Read the model definition and answer for the solid it produces. Units are mm, in the model's axes. Face numbers are marked on the shaded views. A direction names the side the tool comes from. Coordinates: 2 decimals unless noted, no trailing zeros. Order: outer loops, then holes, each group sorted by start corner. A loop starts at its lowest first (then second) coordinate and runs counter-clockwise, first axis right, second up. Notation, with made-up numbers: (64.25, 49) - (89.25, 49) arc R16 ccw to (89.25, 58) - close; hole circle Ø6 at (-22.5, -0.75). An arc over 180 degrees is marked (long way). Write item = value, one per line.
from build123d import *

# Parameters (mm, degrees)
F0_W      = 25.4
F0_H      = 25.4
F1_DEPTH  = 76.2
F2_W      = 5.08
F2_H      = 7.62
F3_DEPTH  = 25.4
F4_W      = 76.2
F4_H      = 25.4
F4_W_2    = 71.12
F4_H_2    = 15.24
F5_DEPTH  = 2.54
F6_W      = 76.2
F6_H      = 25.4
F6_W_2    = 71.12
F6_H_2    = 15.24
F7_DEPTH  = 2.54
F8_W      = 5.08
F8_H      = 7.62
F8_W_2    = 2.54
F8_W_3    = 3.81
F9_DEPTH  = 25.4
F10_W     = 7.62
F10_H     = 12.7
F11_DEPTH = 25.4
F12_W     = 2.54
F12_H     = 71.12
F13_DEPTH = 2.54
F14_W     = 71.12
F14_H     = 15.24
F15_DEPTH = 2.54
F16_W     = 12.7
F16_H     = 7.62
F17_DEPTH = 8.89
F18_W     = 12.7
F18_H     = 7.62
F19_DEPTH = 8.89
F20_W     = 12.7
F20_H     = 7.62
F21_DEPTH = 8.89
F22_W     = 20.32
F22_H     = 22.0218
F22_H_2   = 22.013333
F22_H_3   = 22.004867
F23_DEPTH = 20.32
F25_W     = 76.2
F25_H     = 2.54
F26_DEPTH = 2.54
F27_W     = 2.54
F27_H     = 76.2
F28_DEPTH = 2.54


with BuildPart() as f1:
    # F0 (on Front) → F1 (new body)
    with BuildSketch(Plane.XZ):
        with Locations((12.7, 12.7)):
            Rectangle(F0_W, F0_H)
    extrude(amount=F1_DEPTH)

    # F2 (on face) → F3 (cut)
    with BuildSketch(Plane(origin=(0, 0, 0), x_dir=(0, -1, 0), z_dir=(-1, 0, 0))):
        with Locations((7.62, 12.7)):
            Rectangle(F2_W, F2_H)
        with Locations((38.1, 12.7)):
            Rectangle(F2_W, F2_H)
        with Locations((68.58, 12.7)):
            Rectangle(F2_W, F2_H)
    extrude(amount=-F3_DEPTH, mode=Mode.SUBTRACT)

    # F4 (on face) → F5 (join)
    with BuildSketch(Plane(origin=(0, 0, 0), x_dir=(0, -1, 0), z_dir=(-1, 0, 0))):
        with Locations((38.1, 12.7)):
            Rectangle(F4_W, F4_H)
        with Locations((38.1, 12.7)):
            Rectangle(F4_W_2, F4_H_2, mode=Mode.SUBTRACT)
    extrude(amount=F5_DEPTH)

    # F6 (on face) → F7 (join)
    with BuildSketch(Plane.YZ.offset(25.4)):
        with Locations((-38.1, 12.7)):
            Rectangle(F6_W, F6_H)
        with Locations((-38.1, 12.7)):
            Rectangle(F6_W_2, F6_H_2, mode=Mode.SUBTRACT)
    extrude(amount=F7_DEPTH)

    # F8 (on face) → F9 (cut)
    with BuildSketch(Plane(origin=(0, 0, 0), x_dir=(0, -1, 0), z_dir=(-1, 0, 0))):
        with Locations((12.7, 12.7)):
            Rectangle(F8_W, F8_H)
        with Locations((3.81, 12.7)):
            Rectangle(F8_W_2, F8_H)
        with Locations((33.655, 12.7)):
            Rectangle(F8_W_3, F8_H)
        with Locations((42.545, 12.7)):
            Rectangle(F8_W_3, F8_H)
        with Locations((63.5, 12.7)):
            Rectangle(F8_W, F8_H)
        with Locations((72.39, 12.7)):
            Rectangle(F8_W_2, F8_H)
    extrude(amount=-F9_DEPTH, mode=Mode.SUBTRACT)

    # F10 (on face) → F11 (cut)
    with BuildSketch(Plane(origin=(0, 0, 0), x_dir=(1, 0, 0), z_dir=(0, 0, -1))):
        with Locations((12.7, 8.89)):
            Rectangle(F10_W, F10_H)
        with Locations((12.7, 38.1)):
            Rectangle(F10_W, F10_H)
        with Locations((12.7, 67.31)):
            Rectangle(F10_W, F10_H)
    extrude(amount=-F11_DEPTH, mode=Mode.SUBTRACT)

    # F12 (on face) → F13 (join)
    with BuildSketch(Plane(origin=(0, 0, 0), x_dir=(1, 0, 0), z_dir=(0, 0, -1))):
        Polygon((0, 76.2), (0, 73.66), (2.54, 73.66), (22.86, 73.66), (25.4, 73.66), (25.4, 76.2), align=None)
        with Locations((1.27, 38.1)):
            Rectangle(F12_W, F12_H)
        with Locations((24.13, 38.1)):
            Rectangle(F12_W, F12_H)
        Polygon((2.54, 2.54), (0, 2.54), (0, 0), (25.4, 0), (25.4, 2.54), (22.86, 2.54), align=None)
    extrude(amount=F13_DEPTH)

    # F14 (on face) → F15 (join)
    with BuildSketch(Plane(origin=(0, 0, 0), x_dir=(0, -1, 0), z_dir=(-1, 0, 0))):
        with Locations((38.1, 12.7)):
            Rectangle(F14_W, F14_H)
    extrude(amount=F15_DEPTH)

    # F16 (on face) → F17 (join)
    with BuildSketch(Plane.YZ):
        with Locations((-38.1, 12.7)):
            Rectangle(F16_W, F16_H)
    extrude(amount=F17_DEPTH)

    # F18 (on face) → F19 (join)
    with BuildSketch(Plane.YZ):
        with Locations((-67.31, 12.7)):
            Rectangle(F18_W, F18_H)
    extrude(amount=F19_DEPTH)

    # F20 (on face) → F21 (join)
    with BuildSketch(Plane.YZ):
        with Locations((-8.89, 12.7)):
            Rectangle(F20_W, F20_H)
    extrude(amount=F21_DEPTH)

    # F22 (on face) → F23 (cut)
    with BuildSketch(Plane.XY.offset(25.4)):
        with Locations((12.7, -13.5509)):
            Rectangle(F22_W, F22_H)
        with Locations((12.7, -38.108466)):
            Rectangle(F22_W, F22_H_2)
        with Locations((12.7, -62.657567)):
            Rectangle(F22_W, F22_H_3)
    extrude(amount=-F23_DEPTH, mode=Mode.SUBTRACT)

    # F25 (on face) → F26 (join)
    with BuildSketch(Plane(origin=(0, 0, 0), x_dir=(0, -1, 0), z_dir=(-1, 0, 0))):
        with Locations((38.1, -1.27)):
            Rectangle(F25_W, F25_H)
    extrude(amount=F26_DEPTH)

    # F27 (on face) → F28 (join)
    with BuildSketch(Plane(origin=(0, 0, 0), x_dir=(1, 0, 0), z_dir=(0, 0, -1))):
        with Locations((26.67, 38.1)):
            Rectangle(F27_W, F27_H)
    extrude(amount=F28_DEPTH)


solid = f1.part
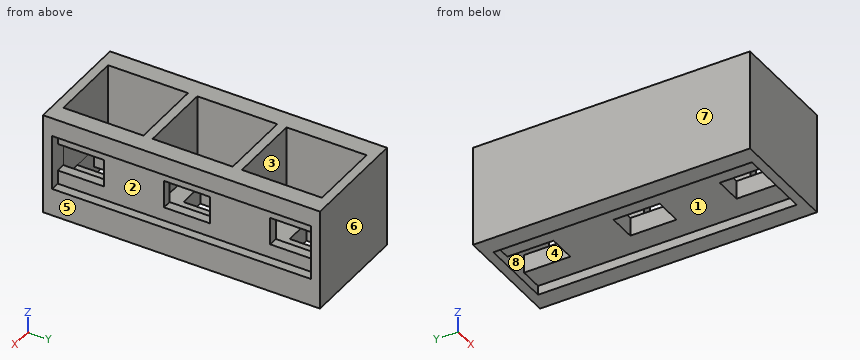
1) The part is cut by section C-C (y = -41). Determine the outline of the cut face in (x, z), and give its area (3 significant figures).
Returned:
outline = (-2.54, -2.54) - (2.54, -2.54) - (2.54, 0) - (8.89, 0) - (8.89, 5.08) - (2.54, 5.08) - (2.54, 25.4) - (-2.54, 25.4) - close; (16.51, 0) - (22.86, 0) - (22.86, -2.54) - (27.94, -2.54) - (27.94, 5.08) - (25.4, 5.08) - (25.4, 8.89) - (22.86, 8.89) - (22.86, 5.08) - (16.51, 5.08) - close; (22.86, 16.51) - (25.4, 16.51) - (25.4, 20.32) - (27.94, 20.32) - (27.94, 25.4) - (22.86, 25.4) - close
area = 290 mm^2
2) The part is cut by section A-A (x = 14.5). Determine the outline of the cut face in (y, z), and give its area (3 significant figures).
Returned:
outline = (-76.2, -2.54) - (-73.66, -2.54) - (-73.66, 25.4) - (-76.2, 25.4) - close; (-60.96, 0) - (-44.45, 0) - (-44.45, 5.08) - (-49.12, 5.08) - (-49.12, 25.4) - (-51.66, 25.4) - (-51.66, 5.08) - (-60.96, 5.08) - close; (-31.75, 0) - (-15.24, 0) - (-15.24, 5.08) - (-24.56, 5.08) - (-24.56, 25.4) - (-27.1, 25.4) - (-27.1, 5.08) - (-31.75, 5.08) - close; (-2.54, -2.54) - (0, -2.54) - (0, 25.4) - (-2.54, 25.4) - close
area = 413 mm^2
3) The part is cut by section D-D (y = -50.5). Determine the outline of the cut face in (x, z), and give its area (3 significant figures).
Returned:
outline = (-2.54, -2.54) - (2.54, -2.54) - (2.54, 0) - (22.86, 0) - (22.86, -2.54) - (27.94, -2.54) - (27.94, 5.08) - (25.4, 5.08) - (25.4, 20.32) - (27.94, 20.32) - (27.94, 25.4) - (-2.54, 25.4) - close
area = 761 mm^2
4) Flat-ended cylindrical pins translate along their axes: pin 1 Ø16.5 at (x, y) = (13, -59.5) entering from +Z; pin 2 Ø6 at (x, y) = (8.5, -12) entering from +Z; pin 3 Ø4.5 at (y, z) = (-33.5, 14) entering from +X; pin 4 Ø2 at (x, y) = (18, -65) entering from -Z. Find the tip coordinate at first contact, or state that the pin passes through.
Returned:
pin_1 = 25.4
pin_2 = 5.08
pin_3 = 25.4
pin_4 = 0
5) For the marked faces 1, 2, 3, 4 and 5, determine the directions among +Z, -Z, +X, -X, +Y, -Y from which every point of the face is accessible in a straight line to the end or side of a thin tool.
Returned:
face_1 = -Z
face_2 = +X
face_3 = +Z
face_4 = +Z, -Z
face_5 = +Z, -Z, +X, +Y, -Y
6) Straight lines are drawn through the part: line 1 along Y through (x, z) = (22.5, 11.75); line 2 along X through (y, z) = (-65, 5); line 3 along X through (y, z) = (-3, -1). For each, find the intervals that lie inside material, in ascending order. Write a range as from..to.
Returned:
line_1 = -76.2..-73.66, -51.66..-49.12, -27.1..-24.56, -2.54..0
line_2 = -2.54..8.89, 16.51..27.94
line_3 = -2.54..2.54, 22.86..27.94
7) Determine the mould class of the marked faces 6, 7 and 8 for opening direction Y: pulls with the +Y half, pulls with the -Y half, needs draft (parallel to the pull), parting line crosses it, or undercut.
Returned:
face_6 = pulls with the +Y half
face_7 = needs draft
face_8 = undercut
8) The part is cut by section B-B (z = 7.75). Determine the outline of the cut face in (x, y), and give its area (3 significant figures).
Returned:
outline = (-2.54, -76.2) - (27.94, -76.2) - (27.94, -73.66) - (25.4, -73.66) - (25.4, -2.54) - (27.94, -2.54) - (27.94, 0) - (-2.54, 0) - close; hole (2.54, -73.66) - (22.86, -73.66) - (22.86, -51.66) - (2.54, -51.66) - close; hole (2.54, -49.12) - (22.86, -49.12) - (22.86, -27.1) - (2.54, -27.1) - close; hole (2.54, -24.56) - (22.86, -24.56) - (22.86, -2.54) - (2.54, -2.54) - close
area = 800 mm^2
